Source: CAD feature listing. Evaluate the final solid. Frame: model axes, mm. Face numbers are marked on the shaded views. Coordinates: 2 decimals unless noted, no trailing zeros. Order: outer loops, then holes, each group sorted by start corner. A loop starts at its lowest first (then second) coordinate and runs counter-clockwise, first axis right, second up.
```python
from build123d import *
from build123d.topology import SkipClean

# Parameters (mm, degrees)
SKETCH_1_W          = 5
SKETCH_1_H          = 10
EXTRUDE_1_DEPTH     = 1
SKETCH_2_W          = 9
SKETCH_2_H          = 1
CUT_EXTRUDE_1_DEPTH = 11.378251298
SKETCH_3_W          = 9
SKETCH_3_H          = 4
EXTRUDE_2_DEPTH     = 9
SKETCH_4_W          = 1
SKETCH_4_H          = 4
EXTRUDE_3_DEPTH     = 1
SKETCH_5_W          = 1
SKETCH_5_H          = 1
EXTRUDE_4_DEPTH     = 1
SKETCH_6_W          = 1
SKETCH_6_H          = 1
EXTRUDE_5_DEPTH     = 1
SKETCH_7_W          = 1
SKETCH_7_H          = 1
EXTRUDE_6_DEPTH     = 1
SKETCH_8_R          = 1
EXTRUDE_7_DEPTH     = 2
CUT_EXTRUDE_START   = -0.5
CUT_EXTRUDE_2_DEPTH = 0.5
EXTRUDE_8_DEPTH     = 0.5
SKETCH_11_R         = 0.3
EXTRUDE_9_DEPTH     = 8
SKETCH_12_R         = 0.3
EXTRUDE_10_DEPTH    = 8
SKETCH_13_R         = 0.3
EXTRUDE_11_DEPTH    = 8


with BuildPart() as part:
    # Эскиз1 → Бобышка-Вытянуть1 (new body)
    with BuildSketch(Plane(origin=(-5, 0, 0), x_dir=(0, -1, 0), z_dir=(-1, 0, 0))):
        with Locations((-0.09, 5)):
            Rectangle(SKETCH_1_W, SKETCH_1_H)
    extrude(amount=-EXTRUDE_1_DEPTH)

    # Эскиз2 → Вырез-Вытянуть1 (cut, through all)
    with BuildSketch(Plane(origin=(-4, 0, 0), x_dir=(0, 0, -1), z_dir=(1, 0, 0))):
        with Locations((-5.5, -1.91)):
            Rectangle(SKETCH_2_W, SKETCH_2_H)
    extrude(amount=-CUT_EXTRUDE_1_DEPTH, mode=Mode.SUBTRACT)

    # Эскиз3 → Бобышка-Вытянуть2 (add)
    with BuildSketch(Plane(origin=(-4, 0, 0), x_dir=(0, 0, -1), z_dir=(1, 0, 0))):
        with Locations((-5.5, 0.59)):
            Rectangle(SKETCH_3_W, SKETCH_3_H)
    extrude(amount=EXTRUDE_2_DEPTH)

    # Эскиз4 → Бобышка-Вытянуть3 (add)
    with BuildSketch(Plane(origin=(0, 0, 1), x_dir=(-1, 0, 0), z_dir=(0, 0, -1))):
        with Locations((-4.5, 0.59)):
            Rectangle(SKETCH_4_W, SKETCH_4_H)
    extrude(amount=EXTRUDE_3_DEPTH)

    # Эскиз5 → Бобышка-Вытянуть4 (add)
    with BuildSketch(Plane.XZ.offset(1.41)):
        with Locations((4.5, 0.5)):
            Rectangle(SKETCH_5_W, SKETCH_5_H)
    extrude(amount=EXTRUDE_4_DEPTH)

    # Эскиз6 → Бобышка-Вытянуть5 (add)
    with BuildSketch(Plane.XZ.offset(1.41)):
        with Locations((-4.5, 9.5)):
            Rectangle(SKETCH_6_W, SKETCH_6_H)
    extrude(amount=EXTRUDE_5_DEPTH)

    # Эскиз7 → Бобышка-Вытянуть6 (add)
    with BuildSketch(Plane.XZ.offset(1.41)):
        with Locations((4.5, 9.5)):
            Rectangle(SKETCH_7_W, SKETCH_7_H)
    extrude(amount=EXTRUDE_6_DEPTH)

    # Эскиз8 → Бобышка-Вытянуть7 (add)
    with BuildSketch(Plane.XY.offset(10)):
        with Locations((-3.8, 1.39)):
            Circle(SKETCH_8_R)
    extrude(amount=EXTRUDE_7_DEPTH)

    # Эскиз9 → Вырез-Вытянуть2 (cut)
    with BuildSketch(Plane.XY.offset(12).offset(CUT_EXTRUDE_START)):
        with BuildLine():
            Line((-4.7367497, 1.04), (-2.8632503, 1.04))
            ThreePointArc((-2.8632503, 1.04), (-3.8, 2.39), (-4.7367497, 1.04))
        make_face()
    extrude(amount=CUT_EXTRUDE_2_DEPTH, mode=Mode.SUBTRACT)

    # Эскиз10 → Бобышка-Вытянуть8 (add)
    with SkipClean():  # the faces are left unmerged after this step: merging them gives an invalid solid
        with BuildSketch(Plane.XY.offset(11.5)):
            with BuildLine():
                Line((-2.8632503, 1.74), (-4.7367497, 1.74))
                ThreePointArc((-4.7367497, 1.74), (-3.8, 2.39), (-2.8632503, 1.74))
            make_face()
        extrude(amount=EXTRUDE_8_DEPTH)

    # Эскиз11 → Бобышка-Вытянуть9 (add)
    with SkipClean():  # the faces are left unmerged after this step: merging them gives an invalid solid
        with BuildSketch(Plane(origin=(0, 0, 1), x_dir=(-1, 0, 0), z_dir=(0, 0, -1))):
            with Locations(Location((-2.54, 0, 0), (0, 0, 180))):
                Circle(SKETCH_11_R)
        extrude(amount=EXTRUDE_9_DEPTH)

    # Эскиз12 → Бобышка-Вытянуть10 (add)
    with SkipClean():  # the faces are left unmerged after this step: merging them gives an invalid solid
        with BuildSketch(Plane(origin=(0, 0, 1), x_dir=(-1, 0, 0), z_dir=(0, 0, -1))):
            with Locations(Location((0, 0, 0), (0, 0, 180))):
                Circle(SKETCH_12_R)
        extrude(amount=EXTRUDE_10_DEPTH)

    # Эскиз13 → Бобышка-Вытянуть11 (add)
    with SkipClean():  # the faces are left unmerged after this step: merging them gives an invalid solid
        with BuildSketch(Plane(origin=(0, 0, 1), x_dir=(-1, 0, 0), z_dir=(0, 0, -1))):
            with Locations(Location((2.54, 0, 0), (0, 0, 180))):
                Circle(SKETCH_13_R)
        extrude(amount=EXTRUDE_11_DEPTH)


solid = part.part
```
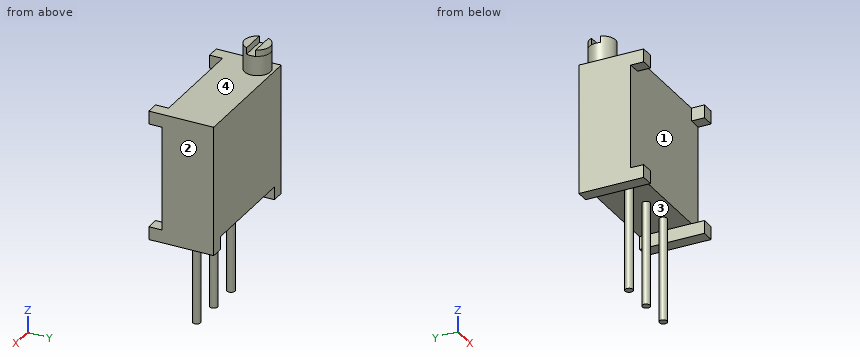
Q1. Pin query (flat end, axial travel): P1, Ø0.8, axis at x = -4.5, y = -2, coming from the +Z side; P2, Ø1.2, axis at x = 1.5, y = 1.5, coming from the -Z side; P3, Ø2.5, axis at x = 2, z = 3.5, coming from the -Y side; P4, Ø0.6, axis at x = -4, y = 1.5, coming from the +Z side. Return the tip coordinate at first contact, or that it passes through.
Solutions:
P1: stops at z = 10
P2: stops at z = 1
P3: stops at y = -1.41
P4: stops at z = 12
Q2. Section query D-D on x = 0. Output: boundary loops of the cut face in (y, z), plus the area to 3 significant figures.
Solutions:
outline: (-1.41, 1) - (-0.3, 1) - (-0.3, -7) - (0.3, -7) - (0.3, 1) - (2.59, 1) - (2.59, 10) - (-1.41, 10) - close
area: 40.8 mm2
Q3. Section query B-B on z = -1.25. Output: boundary loops of the cut face in (x, y), plus the area to 3 significant figures.
Solutions:
outline: circle Ø0.6 at (-2.54, 0); circle Ø0.6 at (0, 0); circle Ø0.6 at (2.54, 0)
area: 0.848 mm2
Q4. Section query C-C on y = -0.95. Output: boundary loops of the cut face in (x, z), plus the area to 3 significant figures.
Solutions:
outline: (-5, 0) - (-4, 0) - (-4, 1) - (4, 1) - (4, 0) - (5, 0) - (5, 10) - (-5, 10) - close
area: 92.0 mm2
Q5. Pull-direction query (Z, two-part tool) for the marked faces 1, 2, 3 and 4; classes: pulls with the +Z half, pulls with the -Z half, needs draft (parallel to the pull), parting line crosses it, or undercut.
Solutions:
face 1: undercut
face 2: needs draft
face 3: pulls with the -Z half
face 4: pulls with the +Z half
Q6. Material intervals for line 1 along X through (y, z) = (-1.65, 0.25); line 2 along Z through (x, y) = (0, -0.75); line 3 along Y through (x, z) = (-1, 2.25), sorted ascending.
Solutions:
line 1: x = -5 to -4, 4 to 5
line 2: z = 1 to 10
line 3: y = -1.41 to 2.59
Q7. Section query A-A on y = -1.8. Output: boundary loops of the cut face in (x, z).
Solutions:
outline: (-5, 0) - (-4, 0) - (-4, 1) - (-5, 1) - close; (-5, 9) - (-4, 9) - (-4, 10) - (-5, 10) - close; (4, 0) - (5, 0) - (5, 1) - (4, 1) - close; (4, 9) - (5, 9) - (5, 10) - (4, 10) - close
